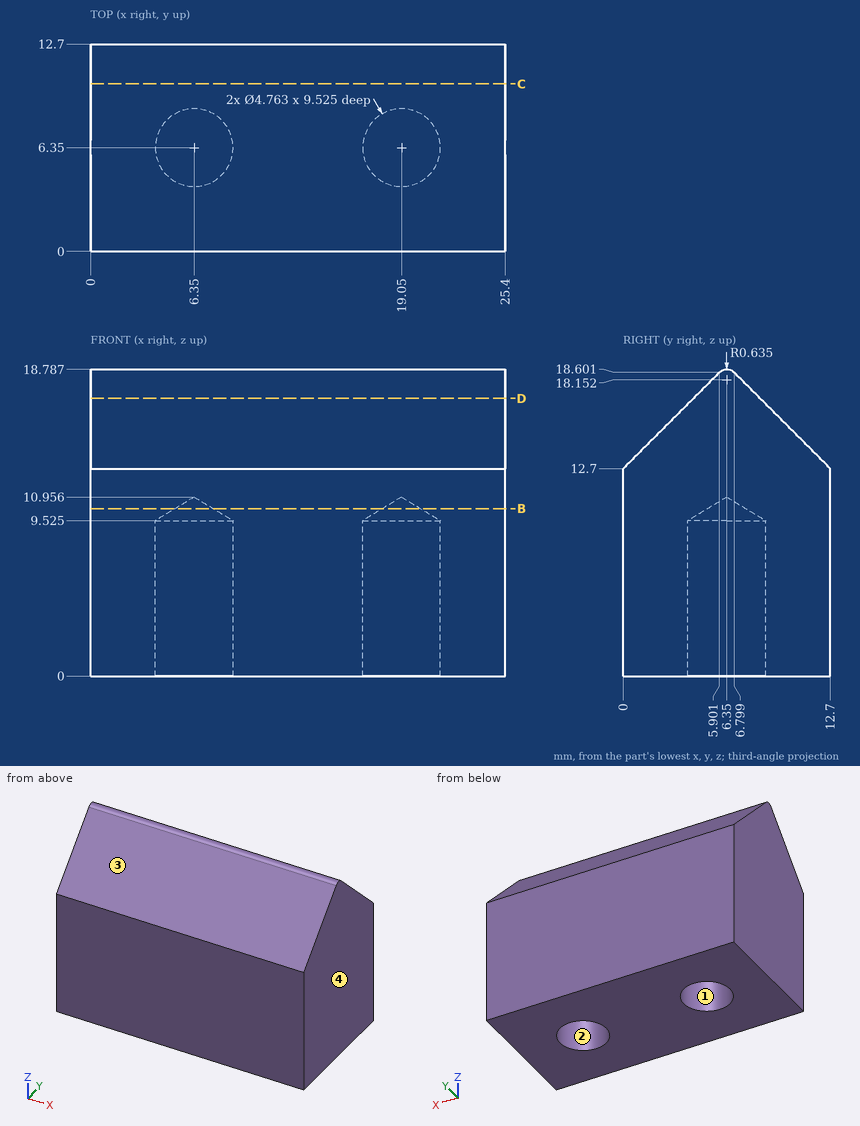
Answer from the drawing. Dimensions are ordinates in mm from the lowest x, y and z of the part. Give positions to 0.01 mm unless a question says otherwise; leave off trailing zeros. Write each loop counter-clockwise with the first axis right and the second up, starting at its lowest first coordinate (ties: lowest second). Pieces come first, ordered by that corner, then holes. Notation, with made-up numbers: (67.25, 37.25) - (71.25, 37.25) arc R15 ccw to (71.25, 41.25) - close; hole circle Ø4 at (-32.5, -6.75). An arc over 180 degrees is marked (long way). One line per item, written item: value. Start each with the question number.
1. Find section C-C (y = 10.25). Write down the section's boundary in (x, z).
2. For a pull along Y with two mould halves and no side action, classify the marked faces 1, 2, 3 and 4 as +Y half, -Y half, draft (parallel to the pull), parting line (faces both ways), or undercut.
3. Find section B-B (z = 10.25). State how many separate pieces and enclosed holes the cut face has, then the cut area to 3 significant figures.
4. Consider probe 1 along Y at (x, z) = (19.05, 4.5); probe 2 along Z at (x, y) = (4.5, 1); probe 3 along Z at (x, y) = (5, 10.5). Determine where each line is inside the solid, lowest interval first.
5. Given pin 1 (3 mm diameter, centred on x = 19.05, y = 6.35, fed in from -Z) (1 decimal); pin 2 (2 mm diameter, centred on x = 22, y = 8.5, fed in from +Z); pin 3 (1.5 mm diameter, centred on x = 4, y = 8.5, fed in from +Z), each flat-ended and moving along its own axis, determine where each tip first touches the part or whether it passes through.
6. Find section D-D (z = 17). Write down the section's boundary in (x, y).
Geometry results:
1. outline: (0, 0) - (25.4, 0) - (25.4, 15.15) - (0, 15.15) - close
2. face 1: undercut
2. face 2: undercut
2. face 3: -Y half
2. face 4: draft
3. separate pieces: 1
3. enclosed holes: 2
3. area: 314 mm2
4. probe 1: 0 to 3.97, 8.73 to 12.7
4. probe 2: 0 to 13.7
4. probe 3: 0 to 14.9
5. pin 1: z = 10.1
5. pin 2: z = 17.9
5. pin 3: z = 17.65
6. outline: (0, 4.3) - (25.4, 4.3) - (25.4, 8.4) - (0, 8.4) - close
